Design review of the part built by this model. Coordinates are the model's own, in mm. A direction names the side the tool comes from. Coordinates: 2 decimals unless noted, no trailing zeros. Loops run counter-clockwise (first coordinate to the right, second up) from the corner with the lowest first, then second, coordinate; pieces in that order, holes last. Notation, with made-up numbers: M 32.25,51.5 L 41.25,51.5 A21 ccw 41.25,64.5 Z; hole C 78,-11.75 d8. An arc over 180 degrees is marked long. Put each result on its own line as item: value. Start each with the question number.
(1) Take a section at D-D, the plane y = -18. Give the boundary of the cut face in (x, z), then the cut area to 3 significant figures.
(2) For faces 4 (the flat face through (4.4, 1.1, 57.9)), 5 (the flat face through (2.5, 3, 24)), 6 (the flat face through (91.049, 34.662, 14.125)), list the 3-axis set-ups (+Z, -Z, +X, -X, +Y, -Y) from which the entire face can be reached by the end or side of a thin tool; tool diameter is ignored.
(3) Take a section at A-A, the plane x = 28.5. Give the boundary of the cut face in (y, z), then the cut area to 3 significant figures.
(4) Take a section at C-C, the plane z = 14.5. Give the boundary of the cut face in (x, y), then the cut area to 3 significant figures.
(5) Clearance check with flat-ended pins moving along their axes: pin 1 (20 mm diameter, centred on y = 28, z = 27.5, fed in from -X); pin 2 (8 mm diameter, centred on x = 87.5, y = 34.5, fed in from +Z); pin 3 (3 mm diameter, centred on x = 8, y = 33.5, fed in from +Z); pin 4 (13.5 mm diameter, centred on x = 69, z = 22, fed in from +Y). State where each tip first meets the part, or that it passes through.
(6) The part is to be moulded in two halves that separate along Y. For faces 1 (the flat face through (48, -22.902, 23)), 2 (the flat face through (97, 3, 25)), 3 (the flat face through (92, 36, 2)), say which applies: +Y half, -Y half, draft (parallel to the pull), parting line (faces both ways), or undercut.
(7) For probe 1 along Y at (x, z) = (54, 5); probe 2 along X at (y, z) = (11, 47); probe 3 along Y at (x, z) = (21, 31.5), list the stretches that pass through material, from the lowest coordinate up. Write a range as [from, to].
(8) Take a section at B-B, the plane y = 7. Give the boundary of the cut face in (x, z), then the cut area to 3 significant figures.
```python
from build123d import *

# Parameters (mm, degrees)
BOSS_EXTRUDE1_DEPTH = 97
SHELL1_T            = -2.5
SKETCH2_W           = 95
SKETCH2_H           = 64
CUT_EXTRUDE1_DEPTH  = 2
BOSS_EXTRUDE2_DEPTH = 93
BOSS_EXTRUDE3_DEPTH = 2
BOSS_EXTRUDE4_DEPTH = 2


with BuildPart() as part:
    # Sketch1 → Boss-Extrude1 (new body)
    with BuildSketch(Plane(origin=(0, 0, 0), x_dir=(0, 0, -1), z_dir=(1, 0, 0))):
        Polygon((0, 41.416666667), (-10, 41.416666667), (-63.911408917, 1.635264119), (-45.805595857, -22.901575437), (0, -22.901575437), align=None)
    extrude(amount=BOSS_EXTRUDE1_DEPTH)

    # Shell1
    shell1_openings = [part.faces().sort_by_distance(p)[0] for p in [
        (48.5, 9.257545615, 0),
        (48.5, 21.525965393, 36.955704458),
    ]]
    offset(amount=SHELL1_T, openings=shell1_openings, kind=Kind.INTERSECTION)

    # Sketch2 → Cut-Extrude1 (cut)
    with BuildSketch(Plane(origin=(0, 31.593177041, 23.312707252), x_dir=(1, 0, 0), z_dir=(0, 0.804647894, 0.593752277))):
        with Locations((48.500142071, -17.236366389)):
            Rectangle(SKETCH2_W, SKETCH2_H)
    extrude(amount=-CUT_EXTRUDE1_DEPTH, mode=Mode.SUBTRACT)

    # Sketch3 → Boss-Extrude2 (add)
    with BuildSketch(Plane.ZY.offset(-94.5)):
        Polygon((11.85497179, 37.56231777), (10.245676001, 38.749822323), (10.36879098, 38.916666667), (6.65116187, 38.916666667), (10.667467236, 35.953021981), align=None)
    extrude(amount=BOSS_EXTRUDE2_DEPTH)

    # Sketch4 → Boss-Extrude3 (add)
    with BuildSketch(Plane(origin=(0, 0, 0), x_dir=(-1, 0, 0), z_dir=(0, 0, -1))):
        Polygon((-94.5, -10.401575437), (-84.5, -20.401575437), (-94.5, -20.401575437), align=None)
        Polygon((-84.5, 38.916666667), (-94.5, 28.916666667), (-94.5, 38.916666667), align=None)
        Polygon((-2.5, 38.916666667), (-2.5, 28.916666667), (-12.5, 38.916666667), align=None)
        Polygon((-2.5, -20.401575437), (-2.5, -10.401575437), (-12.5, -20.401575437), align=None)
    extrude(amount=-BOSS_EXTRUDE3_DEPTH)

    # Sketch5 → Boss-Extrude4 (add)
    with BuildSketch(Plane(origin=(0, 29.983881253, 22.125202698), x_dir=(1, 0, 0), z_dir=(0, 0.804647894, 0.593752277))):
        Polygon((2.5, 12.763633611), (2.5, 5.763633611), (9.5, 12.763633611), align=None)
        Polygon((2.5, -47.955238811), (9.5, -47.955238811), (2.5, -40.955238811), align=None)
        Polygon((94.5, -47.955238811), (94.5, -40.955238811), (87.5, -47.955238811), align=None)
        Polygon((94.5, 12.763633611), (94.5, 5.763633611), (87.5, 12.763633611), align=None)
    extrude(amount=-BOSS_EXTRUDE4_DEPTH)


solid = part.part
```
Computed values:
1. outline: M 0,0 L 10.1,0 L 10.1,2 L 2.5,2 L 2.5,46.32 L 94.5,46.32 L 94.5,2 L 86.9,2 L 86.9,0 L 97,0 L 97,49.42 L 0,49.42 Z
1. area: 563 mm^2
2. face 4: -Z
2. face 5: none
2. face 6: +Z
3. outline: M -22.9,0 L -20.4,0 L -20.4,44.54 L 1.51,60.71 L 0.75,61.74 L 2.36,62.93 L 1.64,63.91 L -22.9,45.81 Z; M 35.95,10.67 L 38.92,6.65 L 38.92,0 L 41.42,0 L 41.42,10 L 40.36,11.43 L 38.75,10.25 L 37.56,11.85 Z
3. area: 219 mm^2
4. outline: M 0,-22.9 L 97,-22.9 L 97,38.1 L 96,38.1 L 96,35.61 L 90.79,35.61 L 92.26,33.12 L 94.5,33.12 L 94.5,-20.4 L 2.5,-20.4 L 2.5,33.12 L 4.74,33.12 L 6.21,35.61 L 1,35.61 L 1,38.1 L 0,38.1 Z
4. area: 542 mm^2
5. pin 1: stops at x = 0
5. pin 2: stops at z = 15.02
5. pin 3: stops at z = 12.89
5. pin 4: stops at y = -20.4
6. face 1: -Y half
6. face 2: draft
6. face 3: undercut
7. probe 1: y = [-22.9, -20.4], [38.92, 41.42]
7. probe 2: x = [0, 2.5], [94.5, 97]
7. probe 3: y = [-22.9, -20.4]
8. outline: M 0,0 L 2.5,0 L 2.5,53.27 L 1,53.27 L 1,56.64 L 0,56.64 Z; M 94.5,0 L 97,0 L 97,56.64 L 96,56.64 L 96,53.27 L 94.5,53.27 Z
8. area: 273 mm^2
